Check sheet for the drawn part. Datum: minimum x, y, z corner. Units: mm. A direction names the side the tool comes from. Coordinates: 2 decimals unless noted, no trailing zeros. Loops run counter-clockwise (first coordinate to the right, second up) from the corner with the lowest first, then second, coordinate; pieces in that order, holes last.
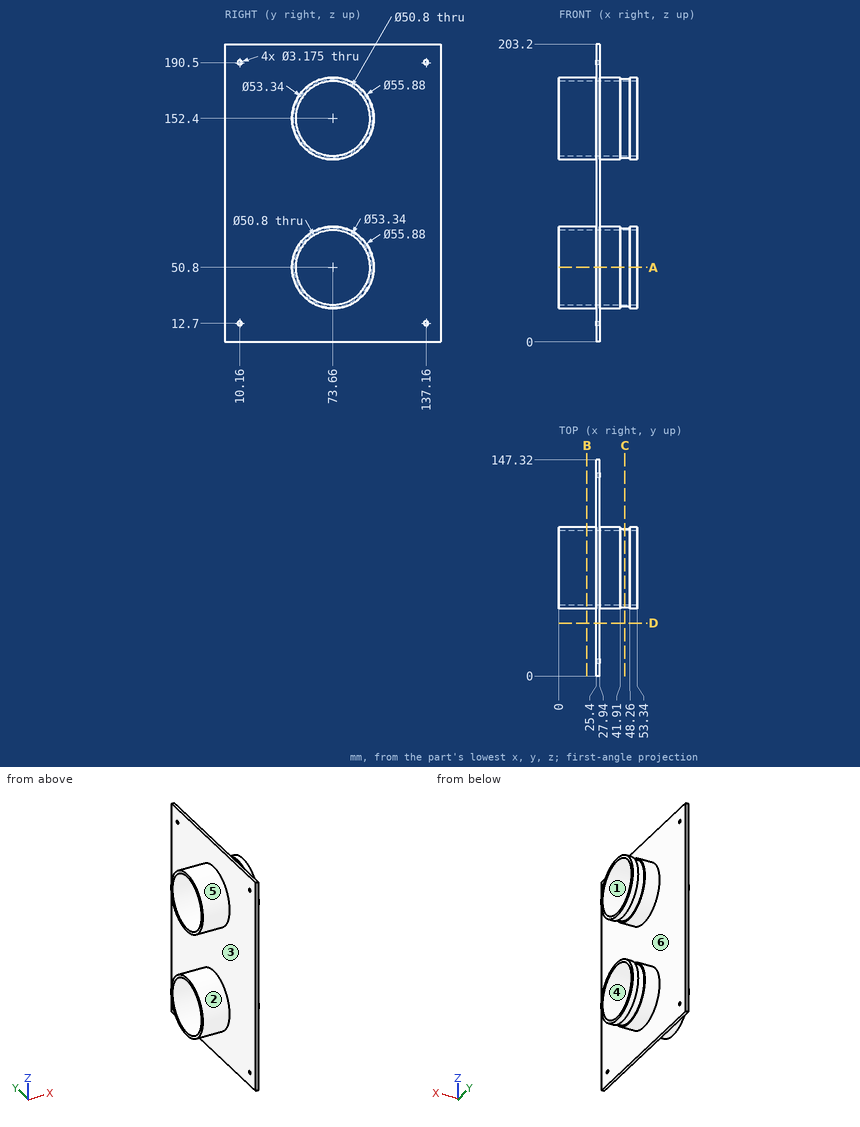
(1) Scan lines: L1, parallel to Y at x = 27.25, z = 12.7; L2, parallel to Z at x = 26, y = 137; L3, parallel to Y at x = 14, z = 152.4. Record each from-to range of solid material in increasing order.
Findings:
L1: y = 0 to 8.57, 11.75 to 135.57, 138.75 to 147.32
L2: z = 0 to 11.12, 14.28 to 188.92, 192.08 to 203.2
L3: y = 45.72 to 48.26, 99.06 to 101.6
(2) Sectioned sample at A-A on z = 50.8. Record the cut outline in (x, y), and give its area (3 significant figures).
Findings:
outline: (0, 45.72) - (25.4, 45.72) - (25.4, 0) - (27.94, 0) - (27.94, 45.72) - (41.91, 45.72) - (41.91, 46.99) - (48.26, 46.99) - (48.26, 45.72) - (53.34, 45.72) - (53.34, 48.26) - (0, 48.26) - close; (0, 99.06) - (53.34, 99.06) - (53.34, 101.6) - (48.26, 101.6) - (48.26, 100.33) - (41.91, 100.33) - (41.91, 101.6) - (27.94, 101.6) - (27.94, 147.32) - (25.4, 147.32) - (25.4, 101.6) - (0, 101.6) - close
area: 487 mm2
(3) Sectioned sample at C-C on x = 45. Record the cut outline in (y, z).
Findings:
outline: circle Ø53.34 at (73.66, 50.8); circle Ø53.34 at (73.66, 152.4); hole circle Ø50.8 at (73.66, 50.8); hole circle Ø50.8 at (73.66, 152.4)
(4) Sectioned sample at B-B on x = 19. Record the cut outline in (y, z).
Findings:
outline: circle Ø55.88 at (73.66, 50.8); circle Ø55.88 at (73.66, 152.4); hole circle Ø50.8 at (73.66, 50.8); hole circle Ø50.8 at (73.66, 152.4)
(5) Gauge pin test, flat ends, axial feed: pin 1 Ø3.5 at (y, z) = (10.16, 12.7) entering from -X; pin 2 Ø4 at (x, z) = (21, 43) entering from +Y; pin 3 Ø3 at (x, y) = (10, 81.5) entering from -Z. Record the tip position at first contact, or that the pin passes through.
Findings:
pin 1: stops at x = 25.4
pin 2: stops at y = 100.99
pin 3: stops at z = 23.59
(6) Sectioned sample at D-D on y = 36. Record the cut outline in (x, z), and give its area (3 significant figures).
Findings:
outline: (25.4, 0) - (27.94, 0) - (27.94, 203.2) - (25.4, 203.2) - close
area: 516 mm2
(7) Access from +Z, -Z, +X, -X, +Y, -Y to the whole of each face (thin tool, end or side, straight path). Record for the marked faces 4, 5 and 6.
Findings:
face 4: +X, -X
face 5: -X
face 6: +X
(8) Draft check along Y on the marked faces 1, 2 and 3. Enter one of: +Y half, -Y half, draft (parallel to the pull), parting line (faces both ways), or undercut.
Findings:
face 1: undercut
face 2: parting line
face 3: draft
